```python
from build123d import *

# Parameters (mm, degrees)
BOSS_EXTRU_1_DEPTH           = 10
ENL_V_MAT_EXTRU_1_DEPTH      = 234.452350599
ENL_V_MAT_EXTRU_1_DEPTH_BACK = 234.452350599
D_GAGEMENT_M51_D             = 5.5


with BuildPart() as part:
    # Esquisse1 → Boss.-Extru.1 (new body)
    with BuildSketch(Plane.XY):
        Polygon((0, 0), (0, 120), (80, 120), (200, 0), align=None)
    extrude(amount=BOSS_EXTRU_1_DEPTH)

    # Esquisse2 → Enlèv. mat.-Extru.1 (cut, two sides: drawn at the far end of the back side and taken through both)
    with BuildSketch(Plane.ZY.offset(-ENL_V_MAT_EXTRU_1_DEPTH_BACK)):
        with BuildLine():
            Line((260.291322683, -16.458785536), (10, 0))
            ThreePointArc((10, 0), (5, 0.164218949), (0, 0))
            Line((0, 0), (-250.291322683, -16.458785536))
            Line((-250.291322683, -16.458785536), (-250.291322683, -518.122568688))
            Line((-250.291322683, -518.122568688), (260.291322683, -518.122568688))
            Line((260.291322683, -518.122568688), (260.291322683, -16.458785536))
        make_face()
    extrude(amount=ENL_V_MAT_EXTRU_1_DEPTH + ENL_V_MAT_EXTRU_1_DEPTH_BACK, mode=Mode.SUBTRACT)

    # Dégagement M51 (through all)
    with Locations(Plane.XY.offset(10)):
        with Locations((155, 14.123808081), (20, 14.123808081)):
            Hole(D_GAGEMENT_M51_D / 2)


solid = part.part
```
Input: part model. Units: mm. Frame: model coordinates. Give positions to 0.01 mm unless a question says otherwise; leave off trailing zeros. Order: outer loops, then holes, each group sorted by start corner. A loop starts at its lowest first (then second) coordinate and runs counter-clockwise, first axis right, second up. Notation, with made-up numbers: M 67,80.25 L 123,80.25 A6 cw 123,88.25 Z; hole C 57,11 d9. An arc over 180 degrees is marked long. One line per question, with ' | ' between items. Start each with the question number.
1. Pull-direction query (Z, two-part tool) for faces 1 (the face through (101.4, 0.164, 5.07)), 2 (the face through (0, 59, 5)), 3 (the face through (79, 48, 0)); classes: released by +Z, released by -Z, zero draft, split by the parting line, or undercut.
2. Section query D-D (z = 7.5). Return the cut outline in (x, y), and give its area (3 significant figures).
3. Section query C-C (x = 20). Return the cut outline in (y, z).
4. Section query B-B (y = 22). Return the cut outline in (x, z), and give its area (3 significant figures).
5. Section query A-A (x = 155). Return the cut outline in (y, z), and give its area (3 significant figures).
6. First-contact query: pin 1 Ø6 at (y, z) = (40, 2) entering from +X; pin 2 Ø1 at (x, z) = (118.5, 5.5) entering from -Y; pin 3 Ø2 at (y, z) = (16, 3) entering from +X. Flat tips, straight axial feed; report the tip coordinate or a pass-through.
7. Material intervals for probe 1 along Y at (x, z) = (20, 7); probe 2 along Y at (x, z) = (155, 5.75); probe 3 along Y at (x, z) = (53.5, 6.25), sorted ascending. Write a range as [from, to].
Here are the results:
1) face 1: undercut | face 2: zero draft | face 3: released by -Z
2) outline: M 0,0.12 L 199.88,0.12 L 80,120 L 0,120 Z; hole C 20,14.12 d5.5; hole C 155,14.12 d5.5 | area: 16,700 mm²
3) outline: M 0,0 L 11.37,0 L 11.37,10 L 0,10 A76.2 cw Z; M 16.87,0 L 120,0 L 120,10 L 16.87,10 Z
4) outline: M 0,0 L 178,0 L 178,10 L 0,10 Z | area: 1,780 mm²
5) outline: M 0,0 L 11.37,0 L 11.37,10 L 0,10 A76.2 cw Z; M 16.87,0 L 45,0 L 45,10 L 16.87,10 Z | area: 394 mm²
6) pin 1: x = 163 | pin 2: y = 0.16 | pin 3: x = 185
7) probe 1: [0.14, 11.37], [16.87, 120] | probe 2: [0.16, 11.37], [16.87, 45] | probe 3: [0.15, 120]
